Design review of the part built by this model. Coordinates are the model's own, in mm. A direction names the side the tool comes from. Round coordinates to 2 decimals unless told otherwise and drop trailing zeros. Loops run counter-clockwise (first coordinate to the right, second up) from the corner with the lowest first, then second, coordinate; pieces in that order, holes last. Notation, with made-up numbers: M 53,38.25 L 99,38.25 A37 cw 99,75.25 Z; hole C -19,28 d3. An arc over 180 degrees is marked long. Use a Markdown table: item, result.
from build123d import *

# Parameters (mm, degrees)
SKETCH2_R           = 16.86788292
SKETCH2_R_2         = 1.697640298
SKETCH2_R_3         = 1.839394333
SKETCH2_R_4         = 1.494089935
BOSS_EXTRUDE1_DEPTH = 12.7


with BuildPart() as part:
    # Sketch2 → Boss-Extrude1 (new body)
    with BuildSketch(Plane.XY):
        Circle(SKETCH2_R)
        with Locations((-9.118891252, 6.145879466)):
            Circle(SKETCH2_R_2, mode=Mode.SUBTRACT)
        with Locations((9.347171253, 3.791989153)):
            Circle(SKETCH2_R_3, mode=Mode.SUBTRACT)
        with Locations((-2.113411396, -11.140283228)):
            Circle(SKETCH2_R_4, mode=Mode.SUBTRACT)
        Polygon((-6.270235486, 3.800984121), (0.156631065, 7.330675279), (6.426866551, 3.529691158), (6.270235486, -3.800984121), (-0.156631065, -7.330675279), (-6.426866551, -3.529691158), align=None, mode=Mode.SUBTRACT)
    extrude(amount=BOSS_EXTRUDE1_DEPTH)


solid = part.part
1. Wall thickness on line 1 along Y through (x, z) = (-1, 2); line 2 along X through (y, z) = (4, 9.5); line 3 along X through (y, z) = (-12.5, 11.75): over which ranges is each line inside the solid? List them lowest first. Write a range as from..to.
Check values:
| item | result |
|---|---|
| line 1 | y = -16.84..-12.14, -10.14..-6.82, 6.7..16.84 |
| line 2 | x = -16.39..-5.91, 5.65..7.52, 11.17..16.39 |
| line 3 | x = -11.33..-2.73, -1.49..11.33 |
2. Take a section at B-B on z = 10. Give the boundary of the cut face in (x, y), and give its area (3 significant figures).
Check values:
| item | result |
|---|---|
| outline | C 0,0 d33.74; hole C -9.12,6.15 d3.4; hole M -6.43,-3.53 L -0.16,-7.33 L 6.27,-3.8 L 6.43,3.53 L 0.16,7.33 L -6.27,3.8 Z; hole C -2.11,-11.14 d2.99; hole C 9.35,3.79 d3.68 |
| area | 727 mm² |
3. The part is to be moulded in two halves that separate along Y. For faces 3 (the face through (7, 0, 12.7)), 4 (the face through (3.1, -5.54, 6.26)), 5 (the face through (-2.196, 16.724, 6.261)), say which applies: pulls with the +Y half, pulls with the -Y half, needs draft (parallel to the pull), parting line crosses it, or undercut.
Check values:
| item | result |
|---|---|
| face 3 | needs draft |
| face 4 | undercut |
| face 5 | parting line crosses it |
4. Insertion check: pin 1 (1.5 mm diameter, centred on y = 3.5, z = 3.5, fed in from -X); pin 2 (1 mm diameter, centred on y = 5.5, z = 4, fed in from +X); pin 3 (4 mm diameter, centred on y = -10, z = 2.5, fed in from +X); pin 4 (3 mm diameter, centred on x = -9.12, y = 6.15, fed in from +Z). Each pin has a flat end and moves straight along its axis. Give the tip position at first contact, or say it passes through.
Check values:
| item | result |
|---|---|
| pin 1 | stops at x = -16.64 |
| pin 2 | stops at x = 16.11 |
| pin 3 | stops at x = 14.85 |
| pin 4 | passes through |
5. Take a section at C-C on y = -4.5. Give the boundary of the cut face in (x, z).
Check values:
| item | result |
|---|---|
| outline | M -16.26,0 L -4.83,0 L -4.83,12.7 L -16.26,12.7 Z; M 5,0 L 16.26,0 L 16.26,12.7 L 5,12.7 Z |
6. Take a section at D-D on x = 8. Give the boundary of the cut face in (y, z).
Check values:
| item | result |
|---|---|
| outline | M -14.85,0 L 2.54,0 L 2.54,12.7 L -14.85,12.7 Z; M 5.04,0 L 14.85,0 L 14.85,12.7 L 5.04,12.7 Z |
7. Machinability: for faces 1 (the face through (-3.248, -5.457, 6.261)), 2 (the face through (7, 0, 0)), which of the approach directions +Z, -Z, +X, -X, +Y, -Y give a long, thin tool a straight path to every point of the face, cutting with its end or side? Answer none if there is none.
Check values:
| item | result |
|---|---|
| face 1 | +Z, -Z |
| face 2 | -Z, +X, -X, +Y, -Y |
8. Take a section at A-A on x = -3. Give the boundary of the cut face in (y, z), and give its area (3 significant figures).
Check values:
| item | result |
|---|---|
| outline | M -16.6,0 L -12.34,0 L -12.34,12.7 L -16.6,12.7 Z; M -9.94,0 L -5.61,0 L -5.61,12.7 L -9.94,12.7 Z; M 5.6,0 L 16.6,0 L 16.6,12.7 L 5.6,12.7 Z |
| area | 249 mm² |
